```python
from build123d import *

# Parameters (mm, degrees)
F0_R      = 1.1
F1_DEPTH  = 1
F2_W      = 6.3
F2_H      = 11.95
F3_DEPTH  = 4.5
F4_DEPTH  = 3
F5_R      = 1.75
F6_DEPTH  = 2
F7_W      = 13.12
F7_H      = 5
F7_H_2    = 1
F8_DEPTH  = 12
F9_W      = 13.12
F9_H      = 5
F9_H_2    = 1
F10_DEPTH = 12


with BuildPart() as f1:
    # F0 (on Top) → F1 (new body)
    with BuildSketch(Plane.XY):
        Polygon((92.88, 0), (92.88, 26.1), (56.46, 26.1), (56.46, 29.9), (46.66, 29.9), (46.66, 26.1), (39.26, 26.1), (39.26, 29.9), (37.11, 29.9), (37.11, 18.3), (23.99, 18.3), (23.99, 28.9), (18.5, 28.9), (18.5, 18.3), (5.38, 18.3), (5.38, 29.9), (0.95, 29.9), (0.95, 26.6), (0, 26.6), (0, 0), align=None)
        with Locations((3.5, 13.75)):
            Circle(F0_R, mode=Mode.SUBTRACT)
        with Locations((45, 12.31)):
            Circle(F0_R, mode=Mode.SUBTRACT)
    extrude(amount=F1_DEPTH)

    # F2 (on face) → F3 (join)
    with BuildSketch(Plane.XY.offset(1)):
        with Locations((51.6, 23.925000114)):
            Rectangle(F2_W, F2_H)
    extrude(amount=F3_DEPTH)

    # F2 (on face) → F4 (join)
    with BuildSketch(Plane.XY.offset(1)):
        Polygon((87.1, 2.400000114), (87.1, 19.150000114), (60.5, 19.150000114), (60.5, 10.150000114), (62.8, 7.700000114), (62.8, 2.400000114), align=None)
    extrude(amount=F4_DEPTH)

    # F5 (on face) → F6 (join)
    with BuildSketch(Plane(origin=(0, 29.9, 0), x_dir=(-1, 0, 0), z_dir=(0, 1, 0))):
        with BuildLine():
            ThreePointArc((-50.5102752641, 1), (-49.4817091985, 1.9222786135), (-49.1, 3.25))
            ThreePointArc((-49.1, 3.25), (-49.4817091985, 4.5777213865), (-50.5102752641, 5.5))
            Line((-50.5102752641, 5.5), (-52.6897247359, 5.5))
            ThreePointArc((-52.6897247359, 5.5), (-54.1, 3.25), (-52.6897247359, 1))
            Line((-52.6897247359, 1), (-50.5102752641, 1))
        make_face()
        with Locations((-51.6, 3.25)):
            Circle(F5_R, mode=Mode.SUBTRACT)
        with BuildLine():
            Line((-52.6897247359, 5.5), (-50.5102752641, 5.5))
            ThreePointArc((-50.5102752641, 5.5), (-51.6, 5.75), (-52.6897247359, 5.5))
        make_face()
        with BuildLine():
            ThreePointArc((-52.6897247359, 1), (-51.6, 0.75), (-50.5102752641, 1))
            Line((-50.5102752641, 1), (-52.6897247359, 1))
        make_face()
    extrude(amount=F6_DEPTH)

    # F7 (on face) → F8 (join)
    with BuildSketch(Plane(origin=(0, 18.3, 0), x_dir=(-1, 0, 0), z_dir=(0, 1, 0))):
        with Locations((-11.94, 3.5)):
            Rectangle(F7_W, F7_H)
        with Locations((-11.94, 0.5)):
            Rectangle(F7_W, F7_H_2)
    extrude(amount=F8_DEPTH)

    # F9 (on face) → F10 (join)
    with BuildSketch(Plane(origin=(0, 18.3, 0), x_dir=(-1, 0, 0), z_dir=(0, 1, 0))):
        with Locations((-30.55, 3.5)):
            Rectangle(F9_W, F9_H)
        with Locations((-30.55, 0.5)):
            Rectangle(F9_W, F9_H_2)
    extrude(amount=F10_DEPTH)


solid = f1.part
```
Part model, mm, in its own coordinate system. A direction names the side the tool comes from. Round coordinates to 2 decimals unless told otherwise and drop trailing zeros. Write each loop counter-clockwise with the first axis right and the second up, starting at its lowest first coordinate (ties: lowest second). Pieces come first, ordered by that corner, then holes. Notation, with made-up numbers: M 0,61.5 L 53,61.5 A12 ccw 53,79.5 Z; hole C 3,67 d11. An arc over 180 degrees is marked long. Answer as CSV lines item,"result". Start each with the question number.
1) Which spindle directions (+Z, -Z, +X, -X, +Y, -Y) get a long thin tool onto all of the face, cutting with end or side? Do faces 1 (the face through (52, 24, 5.5)), 2 (the face through (31, 18.3, 4)), 3 (the face through (53.35, 30.89, 3.33)), 4 (the face through (48.45, 24, 3)), 5 (the face through (12, 30.3, 3)). Say none if no direction does.
2) Drop flat-ended pins along their axis: pin 1 (0.5 mm diameter, centred on x = 0.5, z = 0.5, fed in from +Y); pin 2 (1.5 mm diameter, centred on x = 28.5, z = 2.5, fed in from -Y); pin 3 (2 mm diameter, centred on x = 51, z = 2.5, fed in from -Y). Give the stop position or say it passes through.
3) Drill centre lines: L1, parallel to X at y = 26, z = 1.05; L2, parallel to Z at x = 51.6, y = 31.25; L3, parallel to Y at x = 45, z = 0.35. Where is each one in solid material? Low to high.
4) Band-saw the part on C-C (y = 16.5). List the corners of the cut face in (x, z), then the cut area to 3 significant figures.
5) Mould opens along X. For faces 6 (the face through (75, 2.4, 2)), 7 (the face through (18.5, 24, 3)), 8 (the face through (87.1, 11, 2)) say: +X half, -X half, draft (parallel to the pull), parting line (faces both ways), or undercut.
6) Band-saw the part on B-B (y = 27.5). List the corners of the cut face in (x, z).
7) Band-saw the part on D-D (x = 3.5). List the corners of the cut face in (y, z).
8) Band-saw the part on A-A (x = 45). List the corners of the cut face in (y, z).
Worked out:
1,face 1,"+Z, +X, -Y"
1,face 2,"+Z, -X, -Y"
1,face 3,"+Y"
1,face 4,"+Z, +Y, -Y"
1,face 5,"+Z, -Z, -X, +Y"
2,pin 1,"y = 26.6"
2,pin 2,"y = 18.3"
2,pin 3,"y = 17.95"
3,L1,"5.38 to 18.5, 23.99 to 37.11, 48.45 to 54.75"
3,L2,"0.75 to 1.5, 5 to 5.75"
3,L3,"0 to 11.21, 13.41 to 26.1"
4,outline,"M 0,0 L 92.88,0 L 92.88,1 L 87.1,1 L 87.1,4 L 60.5,4 L 60.5,1 L 0,1 Z"
4,area,"173 mm²"
5,face 6,"draft"
5,face 7,"undercut"
5,face 8,"+X half"
6,outline,"M 0.95,0 L 39.26,0 L 39.26,1 L 37.11,1 L 37.11,6 L 23.99,6 L 23.99,1 L 18.5,1 L 18.5,6 L 5.38,6 L 5.38,1 L 0.95,1 Z; M 46.66,0 L 56.46,0 L 56.46,1 L 54.75,1 L 54.75,5.5 L 48.45,5.5 L 48.45,1 L 46.66,1 Z"
7,outline,"M 0,0 L 12.65,0 L 12.65,1 L 0,1 Z; M 14.85,0 L 29.9,0 L 29.9,1 L 14.85,1 Z"
8,outline,"M 0,0 L 11.21,0 L 11.21,1 L 0,1 Z; M 13.41,0 L 26.1,0 L 26.1,1 L 13.41,1 Z"
